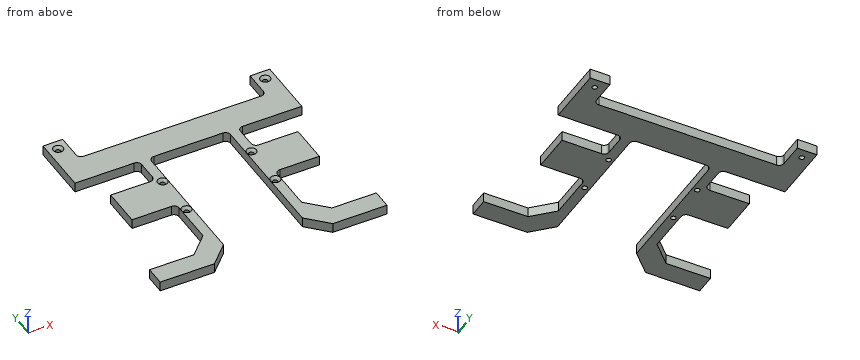
Solid Edge part; units mm, degrees
sketch "Sketch1" plane through (0, 0, 0) normal (0, 0, 1) x (1, 0, 0)
  line L0 (-146.05, 139.7) -> (-146.05, -139.7)
  line L1 (-146.05, -139.7) -> (146.05, -139.7)
  line L2 (146.05, -139.7) -> (146.05, 139.7)
  line L3 (146.05, 139.7) -> (-146.05, 139.7)
  dimension "D1" = 146.05
  dimension "D2" = 146.05
extrude "Protrusion1" add sketch "Sketch1" along normal blind 12.7
sketch "Sketch2" plane through (0, 0, 12.7) normal (0, 0, 1) x (1, 0, 0)
  line L0 (-50.8, -139.7) -> (-50.8, 63.5)
  line L1 (-50.8, 63.5) -> (50.8, 63.5)
  line L2 (50.8, 63.5) -> (50.8, -139.7)
  line L3 (50.8, -139.7) -> (-50.8, -139.7)
  dimension "D1" = 50.8
  dimension "D2" = 50.8
extrude "Cutout1" cut sketch "Sketch2" against normal up to next
sketch "Sketch3" plane through (0, 0, 12.7) normal (0, 0, 1) x (1, 0, 0)
  line L0 (146.05, 38.1) -> (146.05, -38.1)
  line L1 (146.05, -38.1) -> (127, -38.1)
  line L2 (127, -38.1) -> (127, 38.1)
  line L3 (127, 38.1) -> (146.05, 38.1)
  line L4 (-146.05, 38.1) -> (-146.05, -38.1)
  line L5 (-146.05, -38.1) -> (-127, -38.1)
  line L6 (-127, -38.1) -> (-127, 38.1)
  line L7 (-127, 38.1) -> (-146.05, 38.1)
  dimension "D1" = 127
  dimension "D2" = 127
  dimension "D3" = 127
extrude "Cutout2" cut sketch "Sketch3" against normal up to next
sketch "Sketch4" plane through (0, 0, 12.7) normal (0, 0, 1) x (1, 0, 0)
  line L0 (120.65, 101.6) -> (-120.65, 101.6)
  line L1 (-120.65, 139.7) -> (-120.65, 101.6)
  line L2 (120.65, 139.7) -> (-120.65, 139.7)
  line L3 (120.65, 139.7) -> (120.65, 101.6)
  line L4 (146.05, -114.3) -> (63.5, -114.3)
  line L5 (63.5, -114.3) -> (63.5, 63.5)
  line L6 (146.05, 63.5) -> (63.5, 63.5)
  line L7 (146.05, 63.5) -> (146.05, 38.1)
  line L8 (146.05, 38.1) -> (127, 38.1)
  line L9 (127, -38.1) -> (127, 38.1)
  line L10 (146.05, -38.1) -> (127, -38.1)
  line L11 (146.05, -38.1) -> (146.05, -114.3)
  line L12 (-146.05, -114.3) -> (-63.5, -114.3)
  line L13 (-63.5, -114.3) -> (-63.5, 63.5)
  line L14 (-146.05, 63.5) -> (-63.5, 63.5)
  line L15 (-146.05, 63.5) -> (-146.05, 38.1)
  line L16 (-146.05, 38.1) -> (-127, 38.1)
  line L17 (-127, -38.1) -> (-127, 38.1)
  line L18 (-146.05, -38.1) -> (-127, -38.1)
  line L19 (-146.05, -38.1) -> (-146.05, -114.3)
extrude "Cutout3" cut sketch "Sketch4" against normal through all
chamfer "Chamfer_1" distance 25.4 angle 45 4 edges at (-63.5, -114.3, 6.35) (-50.8, -139.7, 6.35) (50.8, -139.7, 6.35) (63.5, -114.3, 6.35)
hole "Hole_1" at (-57.15, -38.1, 12.7) direction (0, 0, -1) diameter 6.35 end up to next countersink diameter 12.7 countersink angle 82
hole "Hole1" at (57.15, -38.1, 12.7) direction (0, 0, -1) diameter 6.35 end up to next countersink diameter 12.7 countersink angle 82
hole "Hole2" at (57.15, 19.05, 12.7) direction (0, 0, -1) diameter 6.35 end up to next countersink diameter 12.7 countersink angle 82
hole "Hole3" at (-57.15, 19.05, 12.7) direction (0, 0, -1) diameter 6.35 end up to next countersink diameter 12.7 countersink angle 82
sketch "Sketch5" plane through (0, 0, 12.7) normal (0, 0, 1) x (1, 0, 0)
  line L0 (120.65, 25.4) -> (120.65, -25.4)
  line L1 (120.65, -25.4) -> (63.5, -25.4)
  line L2 (63.5, -25.4) -> (63.5, 25.4)
  line L3 (63.5, 25.4) -> (120.65, 25.4)
  line L4 (-120.65, 25.4) -> (-120.65, -25.4)
  line L5 (-120.65, -25.4) -> (-63.5, -25.4)
  line L6 (-63.5, -25.4) -> (-63.5, 25.4)
  line L7 (-63.5, 25.4) -> (-120.65, 25.4)
  dimension "D1" = 120.65
  dimension "D2" = 120.65
extrude "ExtrudedProtrusion_2" add sketch "Sketch5" against normal blind 12.7
hole "Hole4" at (133.35, 127, 12.7) direction (0, 0, -1) diameter 6.35 end up to next countersink diameter 12.7 countersink angle 82
hole "Hole5" at (-133.35, 127, 12.7) direction (0, 0, -1) diameter 6.35 end up to next countersink diameter 12.7 countersink angle 82
fillet "Round_1" radius 6.35 10 edges at (-63.5, 63.5, 6.35) (-63.5, 25.4, 6.35) (-63.5, -25.4, 6.35) (63.5, 63.5, 6.35) (63.5, 25.4, 6.35) (63.5, -25.4, 6.35) (-50.8, 63.5, 6.35) (50.8, 63.5, 6.35) (-120.65, 101.6, 6.35) (120.65, 101.6, 6.35)
properties part number "CHAS-01"
Check sheet for the modelled part. Datum: model origin and axes. Units: mm. Give positions to 0.01 mm unless a question says otherwise; leave off trailing zeros. Loops run counter-clockwise (first coordinate to the right, second up) from the corner with the lowest first, then second, coordinate; pieces in that order, holes last. Notation, with made-up numbers: M 44,2 L 96,2 A13 ccw 96,27 Z; hole C 67.5,-27 d6. An arc over 180 degrees is marked long. Return JSON: item names as keys, results as strings. Group by question number.
1. Go/stop test with flat-tipped pins: pin 1 (1.5 mm diameter, centred on y = -7.5, z = 7, fed in from +X); pin 2 (8.5 mm diameter, centred on x = 133.35, y = 127, fed in from +Z); pin 3 (5 mm diameter, centred on x = 106, z = 2, fed in from +Y). Record where each tip stops, or that it passes through.
2. Cross-section at B-B on x = -27. Record the boundary of the cut face in (y, z), plus the area to 3 significant figures.
3. Thickness scan on L1, parallel to X at y = -38.1, z = 4.5 (3 decimals); L2, parallel to Y at x = -98, z = 5.5; L3, parallel to Y at x = 57.15, z = 2.75 (3 decimals). Record the ranges inside material, lowest first.
4. Cross-section at A-A on z = 3.5. State how many separate pieces and enclosed holes the cut face has, plus the area to 3 significant figures.
Return value:
{
 "1": {"pin 1": "x = 120.65", "pin 2": "z = 10.28", "pin 3": "y = 101.6"},
 "2": {"outline": "M 63.5,0 L 101.6,0 L 101.6,12.7 L 63.5,12.7 Z", "area": "484 mm^2"},
 "3": {"L1": "-63.5 to -60.325, -53.975 to -50.8, 50.8 to 53.975, 60.325 to 63.5", "L2": "-139.7 to -114.3, -25.4 to 25.4, 63.5 to 101.6", "L3": "-120.65 to -41.275, -34.925 to 15.875, 22.225 to 101.6"},
 "4": {"separate pieces": "1", "enclosed holes": "6", "area": "28,100 mm^2"}
}
